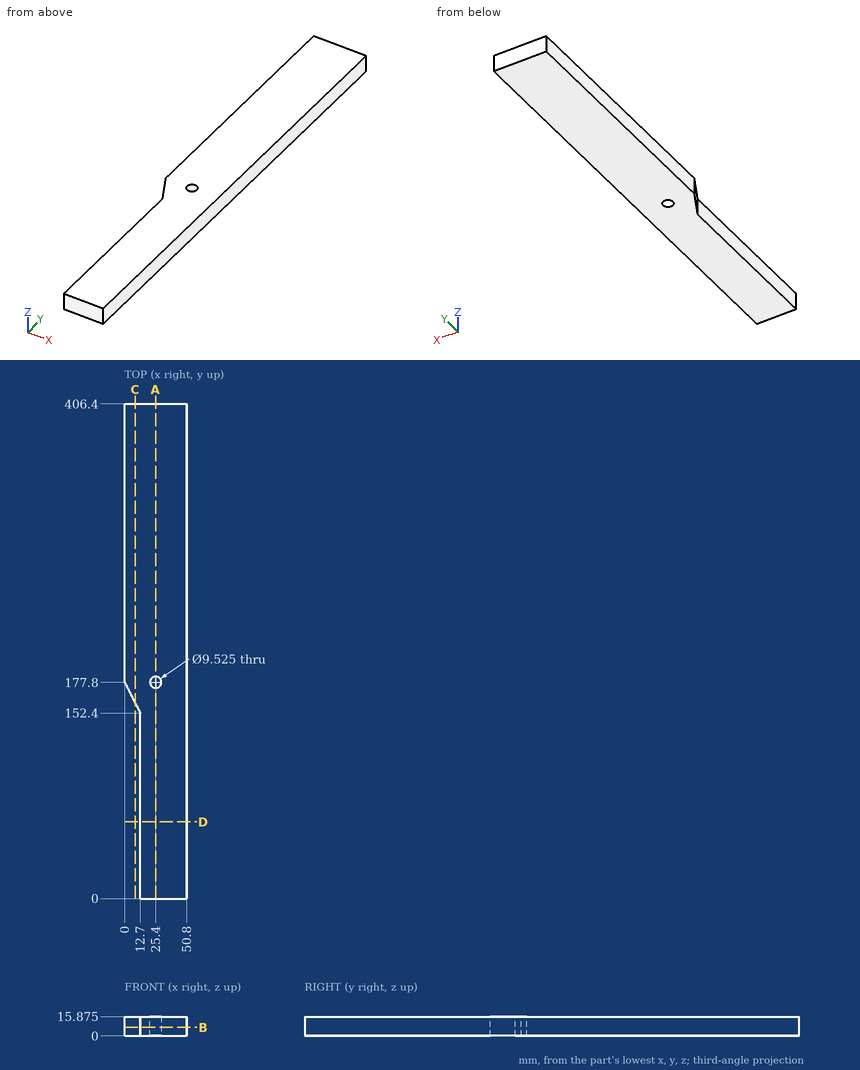
Geometry: see drawing. Coordinates: mm, zero at the bounding-box minimum. Round coordinates to 2 decimals unless told otherwise and drop trailing zeros. Loops run counter-clockwise (first coordinate to the right, second up) from the corner with the lowest first, then second, coordinate; pieces in that order, holes last.
(1) Section query A-A (x = 25.4). Output: boundary loops of the cut face in (y, z) (1 decimal), and give its area (3 significant figures).
From the geometry:
outline: (0, 0) - (173, 0) - (173, 15.9) - (0, 15.9) - close; (182.6, 0) - (406.4, 0) - (406.4, 15.9) - (182.6, 15.9) - close
area: 6,300 mm2
(2) Section query D-D (y = 63). Output: boundary loops of the cut face in (x, z) (3 decimals).
From the geometry:
outline: (12.7, 0) - (50.8, 0) - (50.8, 15.875) - (12.7, 15.875) - close
(3) Section query C-C (x = 8.5). Output: boundary loops of the cut face in (y, z) (3 decimals).
From the geometry:
outline: (160.8, 0) - (406.4, 0) - (406.4, 15.875) - (160.8, 15.875) - close
(4) Section query B-B (z = 7). Output: boundary loops of the cut face in (x, y) (1 decimal).
From the geometry:
outline: (0, 177.8) - (12.7, 152.4) - (12.7, 0) - (50.8, 0) - (50.8, 406.4) - (0, 406.4) - close; hole circle Ø9.5 at (25.4, 177.8)
(5) Material intervals for probe 1 along Y at (x, z) = (25.4, 7.25); probe 2 along X at (y, z) = (119.5, 14.5); probe 3 along Y at (x, z) = (24.5, 8.75), sorted ascending.
From the geometry:
probe 1: y = 0 to 173.04, 182.56 to 406.4
probe 2: x = 12.7 to 50.8
probe 3: y = 0 to 173.12, 182.48 to 406.4
